Verification items for the finished model (mm, model axes). Coordinates: 2 decimals unless noted, no trailing zeros. Order: outer loops, then holes, each group sorted by start corner. A loop starts at its lowest first (then second) coordinate and runs counter-clockwise, first axis right, second up. Notation, with made-up numbers: M 82,21 L 131,21 A22 ccw 131,30 Z; hole C -29.5,-37.75 d7. An arc over 180 degrees is marked long. Return JSON: item names as keys, results as strings. Group by question number.
Q1. Section check B-B, the plane x = 3.75. Enter the section's corners in (y, z) (3 decimals), then the cut area to 3 significant figures.
Q2. Section check A-A, the plane y = -115. Enter the section's corners in (x, z) (3 decimals), then the cut area to 3 significant figures.
Q3. Thickness scan on probe 1 along Z at (x, y) = (7.75, -36.5) (3 decimals); probe 2 along Z at (x, y) = (11.5, -164.5) (3 decimals); probe 3 along X at (y, z) = (-186, 14.5). Record the ranges inside material, lowest first.
Q4. Section check C-C, the plane z = 4.5. Enter the section's corners in (x, y).
Q5. Go/stop test with flat-tipped pins: pin 1 Ø6 at (x, z) = (4, 7) entering from +Y; pin 2 Ø4 at (x, z) = (6.5, 13) entering from +Y; pin 3 Ø5 at (y, z) = (-91, 13) entering from +X. Record where each tip stops, or that it passes through.
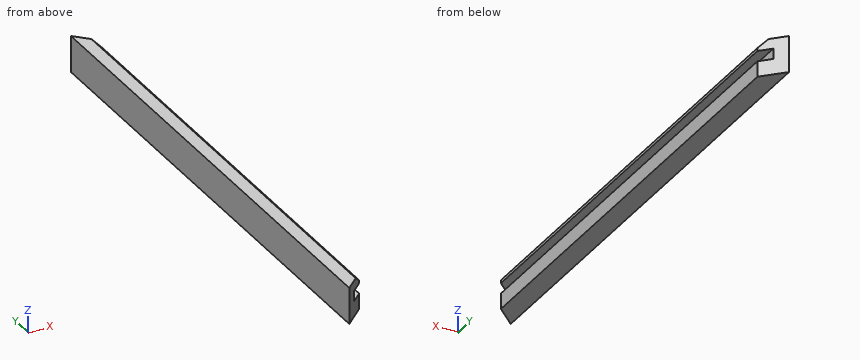
from build123d import *

# Parameters (mm, degrees)
F1_DEPTH = 323.85
F3_DEPTH = 22.226


with BuildPart() as f1:
    # F0 (on Front) → F1 (new body)
    with BuildSketch(Plane.XZ):
        Polygon((0, 22.225), (0, 0), (12.7, 0), (12.7, 9.525), (6.35, 9.525), (6.35, 15.875), (12.7, 15.875), (12.7, 17.734872), (8.209872, 22.225), align=None)
    extrude(amount=F1_DEPTH)

    # F2 (on face) → F3 (cut, through all)
    with BuildSketch(Plane(origin=(0, 0, 0), x_dir=(1, 0, 0), z_dir=(0, 0, -1))):
        Polygon((12.7, 323.85), (0, 323.85), (12.7, 311.15), align=None)
        Polygon((12.7, 12.7), (0, 0), (12.7, 0), align=None)
    extrude(amount=-F3_DEPTH, mode=Mode.SUBTRACT)


solid = f1.part
Numbers:
{
 "1": {"outline": "M -320.1,0 L -3.75,0 L -3.75,22.225 L -320.1,22.225 Z", "area": "7,030 mm2"},
 "2": {"outline": "M 0,0 L 12.7,0 L 12.7,9.525 L 6.35,9.525 L 6.35,15.875 L 12.7,15.875 L 12.7,17.735 L 8.21,22.225 L 0,22.225 Z", "area": "232 mm2"},
 "3": {"probe 1": "z = 0 to 9.525, 15.875 to 22.225", "probe 2": "z = 0 to 9.525, 15.875 to 18.935", "probe 3": "x = 0 to 6.35"},
 "4": {"outline": "M 0,-323.85 L 12.7,-311.15 L 12.7,-12.7 L 0,0 Z"},
 "5": {"pin 1": "stops at y = -1", "pin 2": "stops at y = -4.5", "pin 3": "stops at x = 6.35"}
}
